The model under review builds one solid part; all positions refer to its coordinate system, in mm. Face numbers are marked on the shaded views. A direction names the side the tool comes from. Coordinates: 2 decimals unless noted, no trailing zeros. Write each loop counter-clockwise with the first axis right and the second up, starting at its lowest first coordinate (ties: lowest second). Pieces come first, ordered by that corner, then holes.
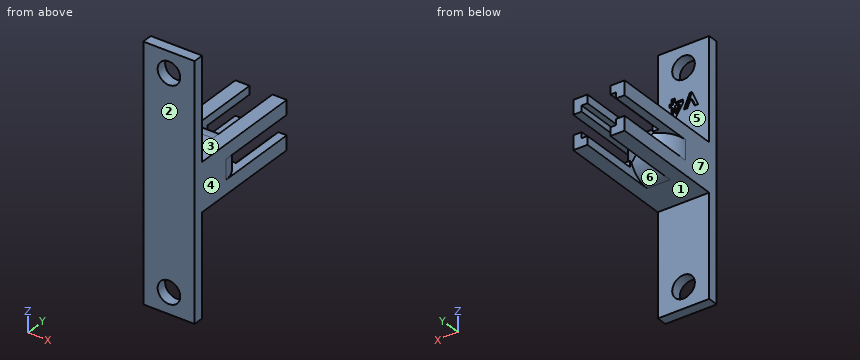
```python
from build123d import *

# Parameters (mm, degrees)
BOSS_EXTRUDE1_DEPTH            = 17.78
BOSS_EXTRUDE1_2_DEPTH          = 17.78
BOSS_EXTRUDE1_3_DEPTH          = 17.78
BOSS_EXTRUDE1_4_DEPTH          = 17.78
SKETCH2_W                      = 15.58
SKETCH2_H                      = 14.58
BOSS_EXTRUDE2_DEPTH            = 17.78
SKETCH3_W                      = 15.58
SKETCH3_H                      = 76.2
SKETCH3_R                      = 3.429
BOSS_EXTRUDE3_DEPTH            = 3.175
CUT_EXTRUDE3_DEPTH             = 0.635
CUT_EXTRUDE4_REACH             = 46.175
CUT_EXTRUDE4_DIRECTION_2_REACH = 46.175
CUT_EXTRUDE5_REACH             = 46.175
CUT_EXTRUDE5_DIRECTION_2_REACH = 46.175


with BuildPart() as part:
    # Sketch1 → Boss-Extrude1 (new body)
    with BuildSketch(Plane(origin=(0, 0, 0), x_dir=(1, 0, 0), z_dir=(0, 1, 0))):
        Polygon((-5.25, 4.75), (-5.25, 2.972), (-7.79, 2.972), (-7.79, 7.29), (-3.472, 7.29), (-3.472, 4.75), align=None)
    extrude(amount=BOSS_EXTRUDE1_DEPTH)



with BuildPart() as body_2:
    # Sketch1 → Boss-Extrude1 2 (new body)
    with BuildSketch(Plane(origin=(0, 0, 0), x_dir=(1, 0, 0), z_dir=(0, 1, 0))):
        Polygon((7.79, 2.972), (7.79, 7.29), (3.472, 7.29), (3.472, 4.75), (5.25, 4.75), (5.25, 2.972), align=None)
    extrude(amount=BOSS_EXTRUDE1_2_DEPTH)


with BuildPart() as body_3:
    # Sketch1 → Boss-Extrude1 3 (new body)
    with BuildSketch(Plane(origin=(0, 0, 0), x_dir=(1, 0, 0), z_dir=(0, 1, 0))):
        Polygon((5.25, -2.972), (7.79, -2.972), (7.79, -7.29), (3.472, -7.29), (3.472, -4.75), (5.25, -4.75), align=None)
    extrude(amount=BOSS_EXTRUDE1_3_DEPTH)


with BuildPart() as body_4:
    # Sketch1 → Boss-Extrude1 4 (new body)
    with BuildSketch(Plane(origin=(0, 0, 0), x_dir=(1, 0, 0), z_dir=(0, 1, 0))):
        Polygon((-5.25, -2.972), (-7.79, -2.972), (-7.79, -7.29), (-3.472, -7.29), (-3.472, -4.75), (-5.25, -4.75), align=None)
    extrude(amount=BOSS_EXTRUDE1_4_DEPTH)


with BuildPart() as part_1:
    add(part.part)

    add(body_2.part)  # Boss-Extrude2 merges body 2

    add(body_3.part)  # Boss-Extrude2 merges body 3

    add(body_4.part)  # Boss-Extrude2 merges body 4
    # Sketch2 → Boss-Extrude2 (add)
    with BuildSketch(Plane(origin=(0, 0, 0), x_dir=(-1, 0, 0), z_dir=(0, -1, 0))):
        Rectangle(SKETCH2_W, SKETCH2_H)
    extrude(amount=BOSS_EXTRUDE2_DEPTH)

    # Sketch3 → Boss-Extrude3 (add)
    with BuildSketch(Plane(origin=(0, -17.78, 0), x_dir=(-1, 0, 0), z_dir=(0, -1, 0))):
        Rectangle(SKETCH3_W, SKETCH3_H)
        with Locations(Location((0, 31.75, 0), (0, 0, 90))):
            Circle(SKETCH3_R, mode=Mode.SUBTRACT)
        with Locations(Location((0, -31.75, 0), (0, 0, 270))):
            Circle(SKETCH3_R, mode=Mode.SUBTRACT)
    extrude(amount=BOSS_EXTRUDE3_DEPTH)

    # Sketch5 → Cut-Extrude3 (cut)
    # profile 1 of 2: a face of its own
    with BuildSketch(Plane(origin=(0, -17.78, 0), x_dir=(1, 0, 0), z_dir=(0, 1, 0))):
        Polygon((-4.402938034, -19.56265828), (-3.33951656, -19.56265828), (-2.238782051, -22.073125862), (-1.138047543, -19.56265828), (-0.074626068, -19.56265828), (-1.937945713, -23.816344178), (-2.539618389, -23.816344178), align=None)
    # profile 2 of 2: a face of its own
    with BuildSketch(Plane(origin=(0, -17.78, 0), x_dir=(1, 0, 0), z_dir=(0, 1, 0))):
        Polygon((2.604916199, -17.846258707), (3.693990385, -17.846258707), (3.693990385, -21.652188195), (4.216372863, -21.652188195), (4.216372863, -22.622327084), (3.693990385, -22.622327084), (3.693990385, -23.816344178), (2.649225427, -23.816344178), (2.649225427, -22.622327084), (0.186565171, -22.622327084), (0.186565171, -21.564735771), align=None)
        Polygon((2.649225427, -21.652188195), (2.649225427, -19.671099286), (1.360759716, -21.652188195), align=None, mode=Mode.SUBTRACT)
    extrude(amount=-CUT_EXTRUDE3_DEPTH, mode=Mode.SUBTRACT)

    # Cut-Extrude4: up to this face of the body (flat: up to its plane)
    cut_extrude4_end = Plane(part_1.part.faces().sort_by_distance((-3.472, 8.89, 6.02))[0])
    # Sketch6 → Cut-Extrude4 (cut, up to the picked face)
    with BuildSketch(Plane(origin=(0, 0, 0), x_dir=(0, 0, -1), z_dir=(1, 0, 0)), mode=Mode.PRIVATE) as cut_extrude4_sk1:
        with BuildLine():
            Line((-7.29, -7.29), (-7.29, 2.54))
            Line((-7.29, 2.54), (7.29, 2.54))
            Line((7.29, 2.54), (7.29, -7.29))
            ThreePointArc((7.29, -7.29), (0, 0), (-7.29, -7.29))
        make_face()
    cut_extrude4_tool1 = split(extrude(cut_extrude4_sk1.sketch, amount=-CUT_EXTRUDE4_REACH, mode=Mode.PRIVATE), bisect_by=cut_extrude4_end, keep=Keep.BOTH, mode=Mode.PRIVATE)
    add(cut_extrude4_tool1.solids().sort_by(Axis((0, 0.165267, 0), (-1, 0, 0)))[0], mode=Mode.SUBTRACT)

    # Cut-Extrude4 direction 2: up to this face of the body (flat: up to its plane)
    cut_extrude4_direction_2_end = Plane(part_1.part.faces().sort_by_distance((3.472, 8.89, 6.02))[0])
    # Sketch6 → Cut-Extrude4 direction 2 (cut, up to the picked face)
    with BuildSketch(Plane(origin=(0, 0, 0), x_dir=(0, 0, -1), z_dir=(1, 0, 0)), mode=Mode.PRIVATE) as cut_extrude4_direction_2_sk1:
        with BuildLine():
            Line((-7.29, -7.29), (-7.29, 2.54))
            Line((-7.29, 2.54), (7.29, 2.54))
            Line((7.29, 2.54), (7.29, -7.29))
            ThreePointArc((7.29, -7.29), (0, 0), (-7.29, -7.29))
        make_face()
    cut_extrude4_direction_2_tool1 = split(extrude(cut_extrude4_direction_2_sk1.sketch, amount=CUT_EXTRUDE4_DIRECTION_2_REACH, mode=Mode.PRIVATE), bisect_by=cut_extrude4_direction_2_end, keep=Keep.BOTH, mode=Mode.PRIVATE)
    add(cut_extrude4_direction_2_tool1.solids().sort_by(Axis((0, 0.165267, 0), (1, 0, 0)))[0], mode=Mode.SUBTRACT)

    # Cut-Extrude5: up to this face of the body (flat: up to its plane)
    cut_extrude5_end = Plane(part_1.part.faces().sort_by_distance((-6.52, 8.89, -2.972))[0])
    # Sketch7 → Cut-Extrude5 (cut, up to the picked face)
    with BuildSketch(Plane.XY, mode=Mode.PRIVATE) as cut_extrude5_sk1:
        with BuildLine():
            Line((-7.79, -7.79), (-7.79, 4.538671937))
            Line((-7.79, 4.538671937), (7.79, 4.538671937))
            Line((7.79, 4.538671937), (7.79, -7.79))
            ThreePointArc((7.79, -7.79), (0, 0), (-7.79, -7.79))
        make_face()
    cut_extrude5_tool1 = split(extrude(cut_extrude5_sk1.sketch, amount=-CUT_EXTRUDE5_REACH, mode=Mode.PRIVATE), bisect_by=cut_extrude5_end, keep=Keep.BOTH, mode=Mode.PRIVATE)
    add(cut_extrude5_tool1.solids().sort_by(Axis((0, 1.190075, 0), (0, 0, -1)))[0], mode=Mode.SUBTRACT)

    # Cut-Extrude5 direction 2: up to this face of the body (flat: up to its plane)
    cut_extrude5_direction_2_end = Plane(part_1.part.faces().sort_by_distance((-6.52, 8.89, 2.972))[0])
    # Sketch7 → Cut-Extrude5 direction 2 (cut, up to the picked face)
    with BuildSketch(Plane.XY, mode=Mode.PRIVATE) as cut_extrude5_direction_2_sk1:
        with BuildLine():
            Line((-7.79, -7.79), (-7.79, 4.538671937))
            Line((-7.79, 4.538671937), (7.79, 4.538671937))
            Line((7.79, 4.538671937), (7.79, -7.79))
            ThreePointArc((7.79, -7.79), (0, 0), (-7.79, -7.79))
        make_face()
    cut_extrude5_direction_2_tool1 = split(extrude(cut_extrude5_direction_2_sk1.sketch, amount=CUT_EXTRUDE5_DIRECTION_2_REACH, mode=Mode.PRIVATE), bisect_by=cut_extrude5_direction_2_end, keep=Keep.BOTH, mode=Mode.PRIVATE)
    add(cut_extrude5_direction_2_tool1.solids().sort_by(Axis((0, 1.190075, 0), (0, 0, 1)))[0], mode=Mode.SUBTRACT)


solid = part_1.part
```
Item 1: To check wall thickness, follow line 1 along X through (y, z) = (-19.1, 31.75); line 2 along Z through (x, y) = (-7, 12); line 3 along Y through (x, z) = (-0.75, 11.5) (3 decimals). State the ranges of each line that lie inside material, in increasing order.
Solved:
line 1: x = -7.79 to -3.43, 3.43 to 7.79
line 2: z = -7.29 to -2.97, 2.97 to 7.29
line 3: y = -20.955 to -17.78
Item 2: Take a section at D-D, the plane x = 6.5. Write out the cut boundary in (y, z) (1 decimal).
Solved:
outline: (-21, -38.1) - (-17.8, -38.1) - (-17.8, -7.3) - (17.8, -7.3) - (17.8, -3) - (-3.5, -3) - (-3.5, 3) - (17.8, 3) - (17.8, 7.3) - (-17.8, 7.3) - (-17.8, 38.1) - (-21, 38.1) - close
Item 3: Take a section at B-B, the plane z = 31.75. Write out the cut boundary in (x, y) (3 decimals).
Solved:
outline: (-7.79, -20.955) - (-3.429, -20.955) - (-3.429, -17.78) - (-7.79, -17.78) - close; (3.429, -20.955) - (7.79, -20.955) - (7.79, -17.78) - (3.429, -17.78) - close
Item 4: Machinability: for the marked faces 1, 2 and 3, which of the approach directions +Z, -Z, +X, -X, +Y, -Y give a long, thin tool a straight path to every point of the face, cutting with its end or side? Answer none if there is none.
Solved:
face 1: -Z, +X, -X, +Y
face 2: +Z, -Z, +X, -X, -Y
face 3: +Z, +X, -X, +Y
Item 5: Take a section at C-C, the plane y = -6. Write out the cut boundary in (x, z), plus the area to 3 significant figures.
Solved:
outline: (-7.79, -7.29) - (-3.47, -7.29) - (-3.47, -7.17) - (3.47, -7.17) - (3.47, -7.29) - (7.79, -7.29) - (7.79, -2.97) - (7.58, -2.97) - (7.58, 2.97) - (7.79, 2.97) - (7.79, 7.29) - (3.47, 7.29) - (3.47, 7.17) - (-3.47, 7.17) - (-3.47, 7.29) - (-7.79, 7.29) - (-7.79, 2.97) - (-7.58, 2.97) - (-7.58, -2.97) - (-7.79, -2.97) - close
area: 223 mm2
Item 6: Mouldability with a two-part tool opening along X and no side actions: class the marked faces 4, 5, 6 and 7 as pulls with the +X half, pulls with the -X half, needs draft (parallel to the pull), parting line crosses it, or undercut.
Solved:
face 4: pulls with the +X half
face 5: needs draft
face 6: undercut
face 7: pulls with the -X half
Item 7: For pin 1 (4.5 mm diameter, centred on x = 2.5, z = 21, fed in from +Y); pin 2 (6 mm diameter, centred on x = 0, z = -31.75, fed in from -Y); pin 3 (4.5 mm diameter, centred on x = 2, y = -2, fed in from -Z); pin 4 (0.9 mm diameter, centred on x = 4.5, z = -3.5, fed in from +Y), all flat-tipped, find the tip position at first contact; note any pin that passes through.
Solved:
pin 1: stops at y = -17.78
pin 2: passes through
pin 3: stops at z = -7.29
pin 4: stops at y = 0
Item 8: Take a section at A-A, the plane y = 5.5. Write out the cut boundary in (x, z).
Solved:
outline: (-7.79, -7.29) - (-3.47, -7.29) - (-3.47, -4.75) - (-5.25, -4.75) - (-5.25, -2.97) - (-7.79, -2.97) - close; (-7.79, 2.97) - (-5.25, 2.97) - (-5.25, 4.75) - (-3.47, 4.75) - (-3.47, 7.29) - (-7.79, 7.29) - close; (3.47, -7.29) - (7.79, -7.29) - (7.79, -2.97) - (5.25, -2.97) - (5.25, -4.75) - (3.47, -4.75) - close; (3.47, 4.75) - (5.25, 4.75) - (5.25, 2.97) - (7.79, 2.97) - (7.79, 7.29) - (3.47, 7.29) - close
